Geometry check sheet. Reference: the model listing, model coordinates, mm. Face numbers are marked on the shaded views. A direction names the side the tool comes from. Coordinates: 2 decimals unless noted, no trailing zeros. Loops run counter-clockwise (first coordinate to the right, second up) from the corner with the lowest first, then second, coordinate; pieces in that order, holes last.
from build123d import *

# Parameters (mm, degrees)
SKETCH_1_R               = 12.2
EXTRUDE_1_DEPTH          = 12.5
SKETCH_2_R               = 3
EXTRUDE_2_DEPTH          = 0.7
SKETCH_3_R               = 3.25
EXTRUDE_3_DEPTH          = 1
SKETCH_4_R               = 1
EXTRUDE_4_DEPTH          = 9.2
SKETCH_5_R               = 0.85
CUT_EXTRUDE_1_DEPTH      = 0.35
SKETCH_9_R               = 0.8
EXTRUDE_7_DEPTH          = 0.3
CUT_EXTRUDE_START        = -0.5
SKETCH_10_R              = 3.25
SKETCH_10_R_2            = 1
CUT_EXTRUDE_3_DEPTH      = 0.5
CUT_EXTRUDE_4_DEPTH      = 2
CUT_EXTRUDE_4_DEPTH_BACK = 0.2
SKETCH_11_R              = 0.3


with BuildPart() as part:
    # 草图1 → 凸台-拉伸1 (new body)
    with BuildSketch(Plane.XY):
        Circle(SKETCH_1_R)
    extrude(amount=EXTRUDE_1_DEPTH)

    # 草图2 → 凸台-拉伸2 (add)
    with BuildSketch(Plane.XY.offset(12.5)):
        Circle(SKETCH_2_R)
    extrude(amount=EXTRUDE_2_DEPTH)

    # 草图3 → 凸台-拉伸3 (add)
    with BuildSketch(Plane(origin=(0, 0, 0), x_dir=(-1, 0, 0), z_dir=(0, 0, -1))):
        Circle(SKETCH_3_R)
    extrude(amount=EXTRUDE_3_DEPTH)

    # 草图4 → 凸台-拉伸4 (add)
    with BuildSketch(Plane(origin=(0, 0, -1), x_dir=(-1, 0, 0), z_dir=(0, 0, -1))):
        Circle(SKETCH_4_R)
    extrude(amount=EXTRUDE_4_DEPTH)

    # 草图5 → 切除-拉伸1 (cut)
    with BuildSketch(Plane(origin=(0, 0, 0), x_dir=(-1, 0, 0), z_dir=(0, 0, -1))):
        with Locations((0, 8.25)):
            Circle(SKETCH_5_R)
        with Locations((7.144709581, 4.125)):
            Circle(SKETCH_5_R)
        with Locations((7.144709581, -4.125)):
            Circle(SKETCH_5_R)
        with Locations((0, -8.25)):
            Circle(SKETCH_5_R)
        with Locations((-7.144709581, -4.125)):
            Circle(SKETCH_5_R)
        with Locations((-7.144709581, 4.125)):
            Circle(SKETCH_5_R)
    extrude(amount=-CUT_EXTRUDE_1_DEPTH, mode=Mode.SUBTRACT)

    # 草图9 → 凸台-拉伸7 (add)
    # profile 1 of 2: a face of its own
    with BuildSketch(Plane(origin=(0, 0, 0), x_dir=(-1, 0, 0), z_dir=(0, 0, -1))):
        with BuildLine():
            Line((-1.205654287, 13.55027997), (-1.205654287, 12.14027997))
            add(Edge.make_bspline(
                [(-1.205654287, 12.14027997), (0, 12.25972003), (1.205654287, 12.14027997)],
                knots=[0, 0, 0, 1, 1, 1], degree=2))
            Line((1.205654287, 12.14027997), (1.205654287, 13.55027997))
            add(Edge.make_bspline(
                [(-1.205654287, 13.55027997), (0, 16.646945855), (1.205654287, 13.55027997)],
                knots=[0, 0, 0, 1, 1, 1], degree=2))
        make_face()
        with Locations((0, 13.85)):
            Circle(SKETCH_9_R, mode=Mode.SUBTRACT)
    # profile 2 of 2: a face of its own
    with BuildSketch(Plane(origin=(0, 0, 0), x_dir=(-1, 0, 0), z_dir=(0, 0, -1))):
        with BuildLine():
            Line((1.205654287, -13.55027997), (1.205654287, -12.14027997))
            add(Edge.make_bspline(
                [(-1.205654287, -12.14027997), (0, -12.25972003), (1.205654287, -12.14027997)],
                knots=[0, 0, 0, 1, 1, 1], degree=2))
            Line((-1.205654287, -12.14027997), (-1.205654287, -13.55027997))
            add(Edge.make_bspline(
                [(-1.205654287, -13.55027997), (0, -16.646945855), (1.205654287, -13.55027997)],
                knots=[0, 0, 0, 1, 1, 1], degree=2))
        make_face()
        with Locations((0, -13.85)):
            Circle(SKETCH_9_R, mode=Mode.SUBTRACT)
    extrude(amount=-EXTRUDE_7_DEPTH)

    # 草图10 → 切除-拉伸3 (cut)
    with BuildSketch(Plane(origin=(0, 0, -1), x_dir=(-1, 0, 0), z_dir=(0, 0, -1)).offset(CUT_EXTRUDE_START)):
        Circle(SKETCH_10_R)
        Circle(SKETCH_10_R_2, mode=Mode.SUBTRACT)
    extrude(amount=CUT_EXTRUDE_3_DEPTH, mode=Mode.SUBTRACT)

    # 草图11 → 切除-拉伸4 (cut, two sides: drawn at the far end of the back side and taken through both)
    with BuildSketch(Plane(origin=(-21.214961085, -62.254689725, -57.176272609), x_dir=(0, 0, 1), z_dir=(0.9558895782864368, -0.2937262571228151, 2.460292199088584e-14)).offset(-CUT_EXTRUDE_4_DEPTH_BACK)):
        with Locations(Location((49.842566165, -65.698034164, 0), (0, 0, 90))):
            Circle(SKETCH_11_R)
    extrude(amount=CUT_EXTRUDE_4_DEPTH + CUT_EXTRUDE_4_DEPTH_BACK, mode=Mode.SUBTRACT)


solid = part.part
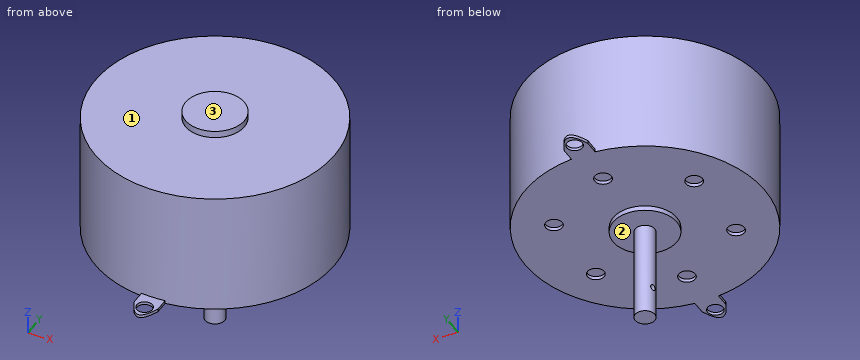
1) Section check B-B on z = 9.5. Record the cut outline in (x, y).
Data:
outline: circle Ø24.4 at (0, 0)
2) Section check C-C on x = 10. Record the cut outline in (y, z).
Data:
outline: (-6.99, 0) - (6.99, 0) - (6.99, 12.5) - (-6.99, 12.5) - close
3) Depth check by flat-ended pin: pin 1 (1.2 mm diameter, centred on x = -0.5, y = -13.5, fed in from +Z); pin 2 (6 mm diameter, centred on x = -0.5, z = -4.5, fed in from -Y); pin 3 (0.5 mm diameter, centred on x = -7, y = -4, fed in from -Z). Enter the tip coordinate at first touch or a pass-through.
Data:
pin 1: stops at z = 0.3
pin 2: stops at y = -1
pin 3: stops at z = 0.35
4) Section check D-D on z = -8.5. Record the cut outline in (x, y).
Data:
outline: circle Ø2 at (0, 0)
5) Section check A-A on y = -8.25. Record the cut outline in (x, z).
Data:
outline: (-8.99, 0) - (-0.85, 0) - (-0.85, 0.35) - (0.85, 0.35) - (0.85, 0) - (8.99, 0) - (8.99, 12.5) - (-8.99, 12.5) - close
6) Access from +Z, -Z, +X, -X, +Y, -Y to the whole of each face (thin tool, end or side, straight path). Record for the marked faces 1, 2 and 3.
Data:
face 1: +Z
face 2: -Z
face 3: +Z, +X, -X, +Y, -Y
7) Material ranges on probe 1 along Y at (x, z) = (0, 0.2); probe 2 along Z at (x, y) = (-6, 2.5); probe 3 along Z at (x, y) = (0.25, 8), recorded low to high.
Data:
probe 1: y = -15.1 to -14.65, -13.05 to -9.1, -7.4 to 7.4, 9.1 to 13.05, 14.65 to 15.1
probe 2: z = 0 to 12.5
probe 3: z = 0.35 to 12.5
